Model file for the job. Use its own axes, mm. Face numbers are marked on the shaded views. A direction names the side the tool comes from. Coordinates: 2 decimals unless noted, no trailing zeros. Write each loop counter-clockwise with the first axis right and the second up, starting at its lowest first coordinate (ties: lowest second). Pieces come first, ordered by that corner, then holes.
Q1. Band-saw the part on B-B, the plane y = 31.75. Write the cut outline in (x, z) (1 decimal).
Q2. Band-saw the part on C-C, the plane z = 133.35. Write the cut outline in (x, y) (3 decimals), plus the area to 3 significant figures.
Q3. Pin check, flat tips, straight feed: P1, Ø7.5, axis at x = 50.8, z = 209.55, coming from the +Y side (3 decimals); P2, Ø10, axis at x = 51.5, y = 14.5, coming from the +Z side. Stop position of each tip, or through.
Q4. Band-saw the part on D-D, the plane x = 12.7. Write the cut outline in (y, z) (3 decimals).
Q5. Pull direction X, two halves, no side cores. Call the marked faces 3, 4 and 5: released by +X, released by -X, zero draft, split by the parting line, or undercut.
Q6. Drill centre lines: probe 1 along Z at (x, y) = (50.8, 2) (3 decimals); probe 2 along Z at (x, y) = (2, 31); probe 3 along X at (y, z) = (11.5, 157.5) (3 decimals). Where is each one in solid material? Low to high.
Q7. Which spindle directions (+Z, -Z, +X, -X, +Y, -Y) get a long thin tool onto all of the face, cutting with end or side? Do the marked faces 1 and 2. Say none if no direction does.
Q8. Band-saw the part on A-A, the plane z = 330.2. Write the cut outline in (x, y) (1 decimal), plus the area to 3 significant figures.
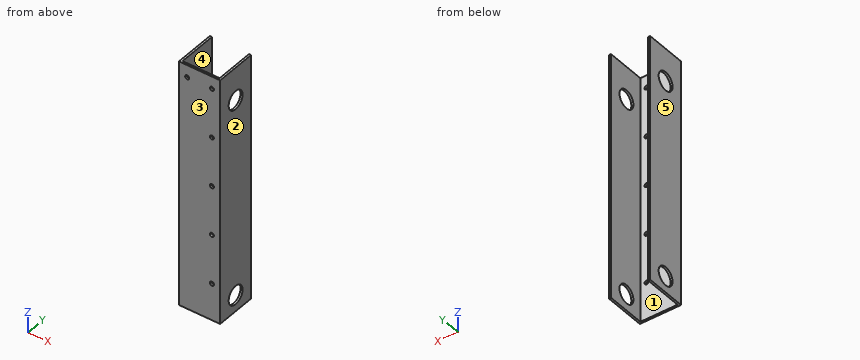
from build123d import *

# Parameters (mm, degrees)
BOSS_EXTRUDE1_DEPTH     = 381
SKETCH2_R               = 3.175
CUT_EXTRUDE1_DEPTH      = 1
CUT_EXTRUDE1_DEPTH_BACK = 64.5
SKETCH3_R               = 14.2875
CUT_EXTRUDE2_DEPTH      = 1
CUT_EXTRUDE2_DEPTH_BACK = 64.5


with BuildPart() as part:
    # Sketch1 → Boss-Extrude1 (new body)
    with BuildSketch(Plane.XY):
        Polygon((0, 0), (63.5, 0), (63.5, 63.5), (60.325, 63.5), (60.325, 3.175), (3.175, 3.175), (3.175, 63.5), (0, 63.5), align=None)
    extrude(amount=BOSS_EXTRUDE1_DEPTH)

    # Sketch2 → Cut-Extrude1 (cut, two sides)
    with BuildSketch(Plane.XZ) as cut_extrude1_sk:
        with Locations((12.7, 361.95)):
            Circle(SKETCH2_R)
        with Locations((50.8, 361.95)):
            Circle(SKETCH2_R)
        with Locations((50.8, 285.75)):
            Circle(SKETCH2_R)
        with Locations((50.8, 209.55)):
            Circle(SKETCH2_R)
        with Locations((50.8, 133.35)):
            Circle(SKETCH2_R)
        with Locations((50.8, 57.15)):
            Circle(SKETCH2_R)
    extrude(amount=CUT_EXTRUDE1_DEPTH, mode=Mode.SUBTRACT)
    extrude(cut_extrude1_sk.sketch, amount=-CUT_EXTRUDE1_DEPTH_BACK, mode=Mode.SUBTRACT)

    # Sketch3 → Cut-Extrude2 (cut, two sides)
    with BuildSketch(Plane(origin=(63.5, 0, 0), x_dir=(0, 0, -1), z_dir=(1, 0, 0))) as cut_extrude2_sk:
        with Locations((-25.4, 31.75)):
            Circle(SKETCH3_R)
        with Locations((-330.2, 31.75)):
            Circle(SKETCH3_R)
    extrude(amount=CUT_EXTRUDE2_DEPTH, mode=Mode.SUBTRACT)
    extrude(cut_extrude2_sk.sketch, amount=-CUT_EXTRUDE2_DEPTH_BACK, mode=Mode.SUBTRACT)


solid = part.part
Answer sheet:
1. outline: (0, 0) - (3.2, 0) - (3.2, 11.1) - (0, 11.1) - close; (0, 39.7) - (3.2, 39.7) - (3.2, 315.9) - (0, 315.9) - close; (0, 344.5) - (3.2, 344.5) - (3.2, 381) - (0, 381) - close; (60.3, 0) - (63.5, 0) - (63.5, 11.1) - (60.3, 11.1) - close; (60.3, 39.7) - (63.5, 39.7) - (63.5, 315.9) - (60.3, 315.9) - close; (60.3, 344.5) - (63.5, 344.5) - (63.5, 381) - (60.3, 381) - close
2. outline: (0, 0) - (47.625, 0) - (47.625, 3.175) - (3.175, 3.175) - (3.175, 63.5) - (0, 63.5) - close; (53.975, 0) - (63.5, 0) - (63.5, 63.5) - (60.325, 63.5) - (60.325, 3.175) - (53.975, 3.175) - close
2. area: 565 mm2
3. P1: stops at y = 3.175
3. P2: passes through
4. outline: (0, 0) - (3.175, 0) - (3.175, 358.775) - (0, 358.775) - close; (0, 365.125) - (3.175, 365.125) - (3.175, 381) - (0, 381) - close
5. face 3: zero draft
5. face 4: undercut
5. face 5: released by -X
6. probe 1: z = 0 to 53.975, 60.325 to 130.175, 136.525 to 206.375, 212.725 to 282.575, 288.925 to 358.775, 365.125 to 381
6. probe 2: z = 0 to 11.13, 39.67 to 315.93, 344.47 to 381
6. probe 3: x = 0 to 3.175, 60.325 to 63.5
7. face 1: +Z, -Z, +Y
7. face 2: +Z, -Z, +X, +Y, -Y
8. outline: (0, 0) - (63.5, 0) - (63.5, 17.5) - (60.3, 17.5) - (60.3, 3.2) - (3.2, 3.2) - (3.2, 17.5) - (0, 17.5) - close; (0, 46) - (3.2, 46) - (3.2, 63.5) - (0, 63.5) - close; (60.3, 46) - (63.5, 46) - (63.5, 63.5) - (60.3, 63.5) - close
8. area: 403 mm2
